Could you check a few things on this model? Use its own coordinates, in mm. Coordinates: 2 decimals unless noted, no trailing zeros. Loops run counter-clockwise (first coordinate to the right, second up) from the corner with the lowest first, then second, coordinate; pieces in that order, holes last.
1) Will this pin go through, and if not, where does the flat tip stop? P1, Ø12.5, axis at x = 92.5, y = 65, coming from the -Z side.
2) Imagine slicing it at C-C on y = 78. Please give me the cut outline in (x, z), plus the area to 3 significant figures.
3) Thinking about a two-plate mould opening in Y: for faces 1 (the face through (66, 130, 5)), 2 (the face through (64, 0, 5)), 3 (the face through (88.45, 68.72, 5.07)), 4 (the face through (64, 66, 10)), which applies, released by +Y, released by -Y, zero draft, split by the parting line, or undercut?
4) If I drill on line 1 along X through (y, z) = (120, 5.75); line 2 along Y through (x, z) = (25, 4); line 3 along X through (y, z) = (77.5, 3), over which ranges is the centre line in solid material (lowest first)?
5) Imagine slicing it at B-B on y = 120. Please give me the cut outline in (x, z), plus the area to 3 significant figures.
6) Imagine slicing it at D-D on z = 7.25. Please give me the cut outline in (x, y).
7) Imagine slicing it at A-A on x = 92.5. Please give me the cut outline in (y, z), plus the area to 3 significant figures.
Autodesk Inventor part; units mm, degrees
ref_plane "YZ Plane" through (0, 0, 0) normal (1, 0, 0) x (0, 1, 0)
ref_plane "XZ Plane" through (0, 0, 0) normal (0, 1, 0) x (-1, 0, 0)
ref_plane "XY Plane" through (0, 0, 0) normal (0, 0, 1) x (1, 0, 0)
sketch "Sketch1" plane through (0, 0, 0) normal (0, 0, 1) x (1, 0, 0)
  line L0 (0, 0) -> (130, 0)
  line L1 (130, 0) -> (130, 130)
  line L2 (130, 130) -> (0, 130)
  line L3 (0, 130) -> (0, 0)
  dimension "d0" = 130
  dimension "d1" = 130
extrude "Extrusion1" add sketch "Sketch1" along normal blind 10
sketch "Sketch2" plane through (0, 0, 10) normal (0, 0, 1) x (1, 0, 0)
  line L0 (130, 130) -> (0, 130)
  line L1 (0, 130) -> (10, 130)
  line L2 (10, 130) -> (10, 20)
  line L3 (0, 0) -> (130, 0)
  line L4 (10, 20) -> (120, 20)
  line L5 (120, 20) -> (120, 130)
  line L6 (120, 130) -> (120, 10)
  line L7 (120, 10) -> (10, 10)
  line L8 (10, 10) -> (10, 120)
  arc A0 (10, 130) -> (10, 123.825) centre (10, 126.9125) ccw
  line L9 (120, 130) -> (120, 120)
  circle A1 centre (120, 120) radius 5
  circle A2 centre (10, 120) radius 5
  circle A3 centre (10, 20) radius 5
  circle A4 centre (120, 20) radius 5
  dimension "d4" = 10
  dimension "d5" = 110
  dimension "d6" = 110
  dimension "d7" = 110
  dimension "d8" = 120
  dimension "d9" = 110
  dimension "d10" = 110
  dimension "d11" = 10
  dimension "d12" = 10
  dimension "d13" = 10
  dimension "d14" = 10
  dimension "d15" = 10
extrude "Extrusion2" cut sketch "Sketch2" against normal blind 10 contours A1 L5 | L5 A1 | A2 L2 | L2 A0 A2 | A0 L2 A2 | A4 L6 L5 | L5 L4 A4 | A3 L4 L2 | L2 L8 A3 | L6 A4 L4 | L4 A3 L8 picked at (9.758, 124.2455) picked at (8.4412, 122.3255)
sketch "Sketch3" plane through (0, 0, 10) normal (0, 0, 1) x (1, 0, 0)
  line L0 (130, 0) -> (130, 130)
  line L1 (130, 0) -> (130, 65)
  line L2 (130, 65) -> (92.5, 65)
  circle A0 centre (92.5, 65) radius 5.5
  point P0 (0, 0)
  dimension "d18" = 65
  dimension "d19" = 37.5
  dimension "d20" = 11
extrude "Extrusion3" cut sketch "Sketch3" against normal through all
sketch "Sketch4" plane through (0, 0, 0) normal (0, 0, -1) x (-1, 0, 0)
  line L0 (0, 130) -> (0, 0)
  line L1 (0, 130) -> (0, 65)
  line L2 (0, 65) -> (-25, 65)
  circle A0 centre (-25, 65) radius 15
  dimension "d23" = 65
  dimension "d24" = 25
  dimension "d25" = 30
extrude "Extrusion4" cut sketch "Sketch4" against normal blind 10
sketch "Sketch5" plane through (0, 0, 0) normal (0, 0, -1) x (-1, 0, 0)
  line L0 (-128.5875, 65.0875) -> (-103.5875, 65.0875)
  circle A0 centre (-103.5875, 65.0875) radius 5.5
  point P0 (0, 0)
  dimension "d28" = 25
  dimension "d29" = 11
extrude "Extrusion5" cut sketch "Sketch5" against normal blind 11
equation "\"d30\" = d29"
properties part number "PARTIMP"
Filled in:
1. P1: stops at z = 0
2. outline: (0, 0) - (17.52, 0) - (17.52, 10) - (0, 10) - close; (32.48, 0) - (130, 0) - (130, 10) - (32.48, 10) - close
2. area: 1,150 mm2
3. face 1: released by +Y
3. face 2: released by -Y
3. face 3: undercut
3. face 4: zero draft
4. line 1: x = 0 to 5, 15 to 115, 125 to 130
4. line 2: y = 0 to 50, 80 to 130
4. line 3: x = 0 to 16.71, 33.29 to 130
5. outline: (0, 0) - (5, 0) - (5, 10) - (0, 10) - close; (15, 0) - (115, 0) - (115, 10) - (15, 10) - close; (125, 0) - (130, 0) - (130, 10) - (125, 10) - close
5. area: 1,100 mm2
6. outline: (0, 0) - (130, 0) - (130, 130) - (0, 130) - close; hole circle Ø10 at (10, 20); hole circle Ø10 at (10, 120); hole circle Ø30 at (25, 65); hole circle Ø11 at (92.5, 65); hole circle Ø11 at (103.59, 65.09); hole circle Ø10 at (120, 20); hole circle Ø10 at (120, 120)
7. outline: (0, 0) - (59.5, 0) - (59.5, 10) - (0, 10) - close; (70.5, 0) - (130, 0) - (130, 10) - (70.5, 10) - close
7. area: 1,190 mm2
